For this review, take the finished solid that the model builds, in its own axes (mm). A direction names the side the tool comes from. Coordinates: 2 decimals unless noted, no trailing zeros. Write each loop counter-clockwise with the first axis right and the second up, starting at its lowest first coordinate (ties: lowest second). Pieces come first, ordered by that corner, then holes.
1) Insertion check: P1, Ø4, axis at y = -33, z = -33.5, coming from the -X side; P2, Ø0.8, axis at x = 16.5, z = 3.5, coming from the -Y side; P3, Ø1.5, axis at x = 0.5, y = -33.5, coming from the +Z side; P4, Ø20.5, axis at x = -0.5, y = -2, coming from the -Z side. Each pin has a flat end and moves straight along its axis. Give the tip position at first contact, or say it passes through.
2) We need section C-C on z = -23.5. Write out the cut boundary in (x, y), then the cut area to 3 significant figures.
3) To check wall thickness, follow line 1 along Y through (x, z) = (18.5, -26); line 2 along Z through (x, y) = (-1.5, -30); line 3 along Y through (x, z) = (-13, -24). State the ranges of each line that lie inside material, in increasing order.
4) We need section B-B on x = 6. Write out the cut boundary in (y, z).
5) We need section A-A on y = -15.5. Write out the cut boundary in (x, z), then the cut area to 3 significant figures.
6) We need section D-D on y = 15.5. Write out the cut boundary in (x, z), then the cut area to 3 significant figures.
7) For faces 1 (the face through (-13, -33, -3)), 2 (the face through (-9, -26, 0)), 3 (the face through (0, -20.5, -22)), 4 (the face through (16, 17.2, 3)), list the 3-axis set-ups (+Z, -Z, +X, -X, +Y, -Y) from which the entire face can be reached by the end or side of a thin tool; tool diameter is ignored.
from build123d import *

# Parameters (mm, degrees)
SKETCH_1_R          = 11
SKETCH_1_R_2        = 1.7
EXTRUDE_1_DEPTH     = 5
EXTRUDE_2_DEPTH     = 4
SKETCH_3_W          = 41
SKETCH_3_H          = 10
EXTRUDE_3_DEPTH     = 45
EXTRUDE_4_DEPTH     = 5
CUT_EXTRUDE_1_DEPTH = 5
SKETCH_6_W          = 6.2
SKETCH_6_H          = 3
CUT_EXTRUDE_2_DEPTH = 5
SKETCH_8_R          = 11.5
CUT_EXTRUDE_3_DEPTH = 5
SKETCH_9_W          = 5
SKETCH_9_H          = 46
EXTRUDE_5_DEPTH     = 5
SKETCH_10_R         = 14
CUT_EXTRUDE_4_DEPTH = 5
SKETCH_11_W         = 20.5
SKETCH_11_H         = 30.5
CUT_EXTRUDE_5_DEPTH = 5
SKETCH_12_W         = 1
SKETCH_12_H         = 5
CUT_EXTRUDE_6_DEPTH = 20
CUT_EXTRUDE_7_DEPTH = 5
EXTRUDE_6_DEPTH     = 1
SKETCH_16_W         = 2
SKETCH_16_H         = 45
SKETCH_16_W_2       = 1.95
EXTRUDE_7_DEPTH     = 5
SKETCH_17_W         = 2
SKETCH_17_H         = 42
SKETCH_17_H_2       = 3
SKETCH_17_W_2       = 6.2
SKETCH_17_W_3       = 9.9
CUT_EXTRUDE_8_DEPTH = 5


with BuildPart() as part:
    # 草图1 → 凸台-拉伸1 (new body)
    with BuildSketch(Plane.XY):
        Polygon((-20.5, 0), (-20.5, -16.5), (-16.5, -20.5), (0, -20.5), (16.5, -20.5), (20.5, -16.5), (20.5, 0), (20.5, 16.5), (16.5, 20.5), (0, 20.5), (-16.5, 20.5), (-20.5, 16.5), align=None)
        Circle(SKETCH_1_R, mode=Mode.SUBTRACT)
        with Locations((15.5, -15.5)):
            Circle(SKETCH_1_R_2, mode=Mode.SUBTRACT)
        with Locations((15.5, 15.5)):
            Circle(SKETCH_1_R_2, mode=Mode.SUBTRACT)
        with Locations((-15.5, 15.5)):
            Circle(SKETCH_1_R_2, mode=Mode.SUBTRACT)
        with Locations((-15.5, -15.5)):
            Circle(SKETCH_1_R_2, mode=Mode.SUBTRACT)
    extrude(amount=EXTRUDE_1_DEPTH)

    # 草图2 → 凸台-拉伸2 (add)
    with BuildSketch(Plane(origin=(0, 0, 0), x_dir=(-1, 0, 0), z_dir=(0, 0, -1))):
        Polygon((-16.5, -30.5), (16.5, -30.5), (20.5, -30.5), (20.5, -16.5), (16.5, -20.5), (-16.5, -20.5), (-20.5, -16.5), (-20.5, -30.5), align=None)
    extrude(amount=-EXTRUDE_2_DEPTH)

    # 草图3 → 凸台-拉伸3 (add)
    with BuildSketch(Plane(origin=(0, 0, 0), x_dir=(-1, 0, 0), z_dir=(0, 0, -1))):
        with Locations((0, -25.5)):
            Rectangle(SKETCH_3_W, SKETCH_3_H)
    extrude(amount=EXTRUDE_3_DEPTH)

    # 草图4 → 凸台-拉伸4 (add)
    with BuildSketch(Plane.XZ.offset(30.5)):
        Polygon((-13.6, -2.908443575), (-13.6, 4), (-7.4, 4), (-7.4, -2.908443575), (-7.4, -45), (-13.6, -45), align=None)
    extrude(amount=EXTRUDE_4_DEPTH)

    # 草图5 → 切除-拉伸1 (cut)
    with BuildSketch(Plane.XY.offset(5)):
        with BuildLine():
            Line((15.5, 17.2), (15.5, 13.8))
            Line((15.5, 13.8), (17.2, 13.8))
            ThreePointArc((17.2, 13.8), (18.9, 15.5), (17.2, 17.2))
            Line((17.2, 17.2), (15.5, 17.2))
        make_face()
        with BuildLine():
            Line((15.5, -13.8), (15.5, -17.2))
            Line((15.5, -17.2), (17.2, -17.2))
            ThreePointArc((17.2, -17.2), (18.9, -15.5), (17.2, -13.8))
            Line((17.2, -13.8), (15.5, -13.8))
        make_face()
        with BuildLine():
            Line((-15.5, -13.8), (-15.5, -17.2))
            Line((-15.5, -17.2), (-13.8, -17.2))
            ThreePointArc((-13.8, -17.2), (-12.1, -15.5), (-13.8, -13.8))
            Line((-13.8, -13.8), (-15.5, -13.8))
        make_face()
        with BuildLine():
            Line((-15.5, 17.2), (-15.5, 13.8))
            Line((-15.5, 13.8), (-13.8, 13.8))
            ThreePointArc((-13.8, 13.8), (-12.1, 15.5), (-13.8, 17.2))
            Line((-13.8, 17.2), (-15.5, 17.2))
        make_face()
    extrude(amount=-CUT_EXTRUDE_1_DEPTH, mode=Mode.SUBTRACT)

    # 草图6 → 切除-拉伸2 (cut)
    with BuildSketch(Plane(origin=(0, -35.5, 0), x_dir=(-1, 0, 0), z_dir=(0, -1, 0))):
        with Locations((10.5, -2.5)):
            Rectangle(SKETCH_6_W, SKETCH_6_H)
    extrude(amount=-CUT_EXTRUDE_2_DEPTH, mode=Mode.SUBTRACT)

    # 草图8 → 切除-拉伸3 (cut)
    with BuildSketch(Plane.XY.offset(5)):
        Circle(SKETCH_8_R)
    extrude(amount=-CUT_EXTRUDE_3_DEPTH, mode=Mode.SUBTRACT)

    # 草图9 → 凸台-拉伸5 (add)
    with BuildSketch(Plane.XZ.offset(30.5)):
        with Locations((2, -22)):
            Rectangle(SKETCH_9_W, SKETCH_9_H)
    extrude(amount=EXTRUDE_5_DEPTH)

    # 草图10 → 切除-拉伸4 (cut)
    with BuildSketch(Plane.XY.offset(5)):
        Circle(SKETCH_10_R)
    extrude(amount=-CUT_EXTRUDE_4_DEPTH, mode=Mode.SUBTRACT)

    # 草图11 → 切除-拉伸5 (cut)
    with BuildSketch(Plane.XY.offset(5)):
        with Locations((-10.25, -15.25)):
            Rectangle(SKETCH_11_W, SKETCH_11_H)
    extrude(amount=-CUT_EXTRUDE_5_DEPTH, mode=Mode.SUBTRACT)

    # 草图12 → 切除-拉伸6 (cut)
    with BuildSketch(Plane.ZY.offset(13.6)):
        with Locations((0.5, -33)):
            Rectangle(SKETCH_12_W, SKETCH_12_H)
    extrude(amount=-CUT_EXTRUDE_6_DEPTH, mode=Mode.SUBTRACT)

    # 草图14 → 切除-拉伸7 (cut)
    with BuildSketch(Plane.XY.offset(5)):
        Polygon((0, -20.5), (10, -30.5), (0, -30.5), align=None)
    extrude(amount=-CUT_EXTRUDE_7_DEPTH, mode=Mode.SUBTRACT)

    # 草图15 → 凸台-拉伸6 (add)
    with BuildSketch(Plane.XY.offset(4)):
        Polygon((0, -20.5), (10, -30.5), (20.5, -30.5), (20.5, -16.5), (16.5, -20.5), align=None)
    extrude(amount=EXTRUDE_6_DEPTH)

    # 草图16 → 凸台-拉伸7 (add)
    with BuildSketch(Plane.XZ.offset(35.5)):
        with Locations((-14.6, -22.5)):
            Rectangle(SKETCH_16_W, SKETCH_16_H)
        with Locations((-1.475, -22.5)):
            Rectangle(SKETCH_16_W_2, SKETCH_16_H)
    extrude(amount=-EXTRUDE_7_DEPTH)

    # 草图17 → 切除-拉伸8 (cut)
    with BuildSketch(Plane.XZ.offset(35.5)):
        with Locations((-8.4, -24)):
            Rectangle(SKETCH_17_W, SKETCH_17_H)
        with Locations((-8.4, -1.5)):
            Rectangle(SKETCH_17_W, SKETCH_17_H_2)
        with Locations((-12.5, -1.5)):
            Rectangle(SKETCH_17_W_2, SKETCH_17_H_2)
        with Locations((-2.45, -1.5)):
            Rectangle(SKETCH_17_W_3, SKETCH_17_H_2)
        with Locations((3.5, -1.5)):
            Rectangle(SKETCH_17_W, SKETCH_17_H_2)
        with Locations((3.5, -24)):
            Rectangle(SKETCH_17_W, SKETCH_17_H)
    extrude(amount=-CUT_EXTRUDE_8_DEPTH, mode=Mode.SUBTRACT)


solid = part.part
Result:
1. P1: stops at x = -15.6
1. P2: stops at y = -30.5
1. P3: stops at z = -3
1. P4: passes through
2. outline: (-20.5, -30.5) - (-15.6, -30.5) - (-15.6, -35.5) - (-9.4, -35.5) - (-9.4, -30.5) - (-2.45, -30.5) - (-2.45, -35.5) - (2.5, -35.5) - (2.5, -30.5) - (20.5, -30.5) - (20.5, -20.5) - (-20.5, -20.5) - close
2. area: 466 mm2
3. line 1: y = -30.5 to -20.5
3. line 2: z = -45 to 0
3. line 3: y = -35.5 to -20.5
4. outline: (-30.5, -45) - (-20.5, -45) - (-20.5, 0) - (-12.65, 0) - (-12.65, 5) - (-26.5, 5) - (-26.5, 0) - (-30.5, 0) - close; (12.65, 0) - (20.5, 0) - (20.5, 5) - (12.65, 5) - close
5. outline: (0, 0) - (13.8, 0) - (13.8, 5) - (0, 5) - close; (18.9, 0) - (20.5, 0) - (20.5, 5) - (18.9, 5) - close
5. area: 77.0 mm2
6. outline: (-20.5, 0) - (-17.2, 0) - (-17.2, 5) - (-20.5, 5) - close; (-12.1, 0) - (13.8, 0) - (13.8, 5) - (-12.1, 5) - close; (18.9, 0) - (20.5, 0) - (20.5, 5) - (18.9, 5) - close
6. area: 154 mm2
7. face 1: +Z, +X, -X, -Y
7. face 2: +Z, -X, -Y
7. face 3: -Z, +X, -X, +Y
7. face 4: +Z, -Z
